Geometry: final body of the model. Coordinates: model frame, mm. A direction names the side the tool comes from. Round coordinates to 2 decimals unless told otherwise and drop trailing zeros. Order: outer loops, then holes, each group sorted by start corner. A loop starts at its lowest first (then second) coordinate and runs counter-clockwise, first axis right, second up. Notation, with made-up numbers: M 68.5,48 L 78.5,48 A15 cw 78.5,71 Z; hole C 75.25,-19.5 d3. An arc over 180 degrees is marked long. Put each result on its own line as item: value. Start each with the question number.
1) First-contact query: P1, Ø8, axis at x = -13, y = 11.5, coming from the +Z side. Flat tip, straight axial feed; report the tip coordinate or a pass-through.
2) Access query for faces 1 (the flat face through (-19.7, 19.8, 19.7)), 2 (the flat face through (2, -2, 42)). Directions: +Z, -Z, +X, -X, +Y, -Y. A direction counts if a zero-diameter tool reaches every point of the face in a straight line with its end or side. Return the directions, or none.
3) Section C-C, the plane z = 20. Return loops of the section in (x, y), then the cut area to 3 significant figures.
4) Material intervals for probe 1 along Z at (x, y) = (20, -13.5); probe 2 along Z at (x, y) = (5, -8.5); probe 3 along Y at (x, z) = (1, 58), sorted ascending. Write a range as [from, to].
5) Section A-A, the plane y = 0. Return loops of the section in (x, z), then the cut area to 4 significant figures.
6) Section D-D, the plane x = -11.5. Return loops of the section in (y, z).
Autodesk Inventor part; units mm, degrees
ref_plane "YZ Plane" through (0, 0, 0) normal (1, 0, 0) x (0, 1, 0)
ref_plane "XZ Plane" through (0, 0, 0) normal (0, 1, 0) x (-1, 0, 0)
ref_plane "XY Plane" through (0, 0, 0) normal (0, 0, 1) x (1, 0, 0)
sketch "Sketch1" plane through (0, 0, 0) normal (0, 0, 1) x (1, 0, 0)
  line L0 (-21.75, -21.75) -> (21.75, -21.75)
  line L1 (21.75, -21.75) -> (21.75, 21.75)
  line L2 (21.75, 21.75) -> (-21.75, 21.75)
  line L3 (-21.75, 21.75) -> (-21.75, -21.75)
  line L4 (-21.75, -21.75) -> (21.75, 21.75) construction
  line L5 (21.75, -21.75) -> (-21.75, 21.75) construction
  point P0 (0, 0)
  dimension "d0" = 43.5
extrude "Extrusion1" add sketch "Sketch1" along normal blind 40
sketch "Sketch2" plane through (0, 0, 40) normal (0, 0, 1) x (1, 0, 0)
  circle A0 centre (0, 0) radius 10
  dimension "d3" = 20
extrude "Extrusion2" add sketch "Sketch2" along normal blind 2
sketch "Sketch3" plane through (0, 0, 42) normal (0, 0, 1) x (1, 0, 0)
  circle A0 centre (0, 0) radius 2.5
  dimension "d6" = 5
extrude "Extrusion3" add sketch "Sketch3" along normal blind 31
chamfer "Chamfer1" distance 4 angle 45 4 edges at (21.75, 21.75, 20) (-21.75, 21.75, 20) (21.75, -21.75, 20) (-21.75, -21.75, 20)
properties part number "Stepper Simulation"
Result sheet:
1. P1: stops at z = 40
2. face 1: +Z, -Z, -X, +Y
2. face 2: +Z
3. outline: M -21.75,-17.75 L -17.75,-21.75 L 17.75,-21.75 L 21.75,-17.75 L 21.75,17.75 L 17.75,21.75 L -17.75,21.75 L -21.75,17.75 Z
3. area: 1,860 mm2
4. probe 1: z = [0, 40]
4. probe 2: z = [0, 42]
4. probe 3: y = [-2.29, 2.29]
5. outline: M -21.75,0 L 21.75,0 L 21.75,40 L 10,40 L 10,42 L 2.5,42 L 2.5,73 L -2.5,73 L -2.5,42 L -10,42 L -10,40 L -21.75,40 Z
5. area: 1,935 mm2
6. outline: M -21.75,0 L 21.75,0 L 21.75,40 L -21.75,40 Z
